Input: part model. Units: mm. Frame: model coordinates. A direction names the side the tool comes from. Give positions to 0.01 mm unless a question says otherwise; leave off trailing zeros. Loops run counter-clockwise (first coordinate to the right, second up) from the corner with the lowest first, then second, coordinate; pieces in that order, holes last. Notation, with made-up numbers: (14, 43.25) -> (50, 43.25) arc R19 ccw to (50, 55.25) -> close; hole circle Ø11 at (31.5, 53). An arc over 180 degrees is marked (long way). Answer as a JSON object with one key per item and string values.
```python
from build123d import *

# Parameters (mm, degrees)
F0_R      = 3.5
F1_DEPTH  = 50
F2_R      = 6
F3_DEPTH  = 150
F4_R      = 20
F5_DEPTH  = 7.9
F6_SIZE   = 1
F7_SIZE   = 0.5
F8_R      = 11
F9_DEPTH  = 3.1
F10_R     = 10
F11_DEPTH = 6
F12_R     = 11
F13_DEPTH = 11
F14_SIZE  = 0.5


with BuildPart() as f1:
    # F0 (on Top) → F1 (new body)
    with BuildSketch(Plane.XY):
        Circle(F0_R)
    extrude(amount=F1_DEPTH)

    # F2 (on face) → F3 (join)
    with BuildSketch(Plane.XY.offset(50)):
        Circle(F2_R)
    extrude(amount=F3_DEPTH)

    # F4 (on face) → F5 (join)
    with BuildSketch(Plane.XY.offset(200)):
        Circle(F4_R)
    extrude(amount=F5_DEPTH)

    # F6
    f6_edges = [f1.edges().sort_by_distance(p)[0] for p in [
        (-6, 0, 50),
    ]]
    chamfer(f6_edges, length=F6_SIZE)

    # F7
    f7_edges = [f1.edges().sort_by_distance(p)[0] for p in [
        (-20, 0, 200),
        (-20, 0, 207.9),
    ]]
    chamfer(f7_edges, length=F7_SIZE)

    # F8 (on face) → F9 (join)
    with BuildSketch(Plane.XY.offset(207.9)):
        Circle(F8_R)
    extrude(amount=F9_DEPTH)

    # F10 (on face) → F11 (join)
    with BuildSketch(Plane.XY.offset(211)):
        Circle(F10_R)
    extrude(amount=F11_DEPTH)

    # F12 (on face) → F13 (join)
    with BuildSketch(Plane.XY.offset(217)):
        Circle(F12_R)
    extrude(amount=F13_DEPTH)

    # F14
    f14_edges = [f1.edges().sort_by_distance(p)[0] for p in [
        (-11, 0, 211),
        (-11, 0, 217),
        (-11, 0, 228),
    ]]
    chamfer(f14_edges, length=F14_SIZE)


solid = f1.part
```
Q1. Section B-B, the plane z = 168.5. Return the cut outline in (x, y), then the cut area to 3 significant figures.
Evaluation:
{"outline": "circle Ø12 at (0, 0)", "area": "113 mm2"}
Q2. Ray query, line 1 along Z through (x, y) = (-6.5, -18); line 2 along Z through (x, y) = (1, 8.5); line 3 along Y through (x, z) = (12, 201.5). Return the intervals inside material, ascending.
Evaluation:
{"line 1": "z = 200 to 207.9", "line 2": "z = 200 to 228", "line 3": "y = -16 to 16"}
Q3. Section A-A, the plane z = 48. Return the cut outline in (x, y), then the cut area to 3 significant figures.
Evaluation:
{"outline": "circle Ø7 at (0, 0)", "area": "38.5 mm2"}
Q4. Access query for faces 1 (the flat face through (5, -9, 211)), 2 (the cylindrical face through (-2.38, -10.74, 209.18)), 3 (the flat face through (4, 5, 200)), 4 (the flat face through (0, 0, 0)). Directions: +Z, -Z, +X, -X, +Y, -Y. A direction counts if a zero-diameter tool reaches every point of the face in a straight line with its end or side. Return the directions, or none.
Evaluation:
{"face 1": "none", "face 2": "+Z", "face 3": "-Z", "face 4": "-Z, +X, -X, +Y, -Y"}
Q5. Draft query along Z for faces 5 (the flat face through (8, -8, 207.9)), 6 (the cylindrical face through (3.233, -1.341, 24.65)), 7 (the flat face through (5, -9, 217)). Return one class per face: +Z half, -Z half, draft (parallel to the pull), parting line (faces both ways), or undercut.
Evaluation:
{"face 5": "+Z half", "face 6": "draft", "face 7": "undercut"}
Q6. Pin query (flat end, axial travel): pin 1 (1 mm diameter, centred on x = -11, y = -15, fed in from +Z); pin 2 (6 mm diameter, centred on x = 1, z = 48.5, fed in from +Y); pin 3 (10 mm diameter, centred on x = -10.5, y = -5, fed in from -Z); pin 4 (10.5 mm diameter, centred on x = -4, y = -5, fed in from -Z). Return the tip coordinate at first contact, or that it passes through.
Evaluation:
{"pin 1": "stops at z = 207.9", "pin 2": "stops at y = 6", "pin 3": "stops at z = 200", "pin 4": "stops at z = 0"}
